Source: CAD feature listing. Evaluate the final solid. Frame: model axes, mm. Face numbers are marked on the shaded views. Round coordinates to 2 decimals unless told otherwise and drop trailing zeros. Order: outer loops, then holes, each group sorted by start corner. A loop starts at its lowest first (then second) coordinate and runs counter-clockwise, first axis right, second up. Notation, with made-up numbers: (-28, -17.75) -> (26, -17.75) arc R4 cw to (26, -10.75) -> close; hole circle Ø3 at (45, -23). An arc over 180 degrees is marked (long way). Write item = value, one per line. Start each with the question number.
(1) Cut plane C-C on x = 0. Return the cut outline in (y, z).
(2) Contact query for a flat-ended pin moving along its axis: pin 1 Ø1.6 at (x, y) = (0, -7.64) entering from -Z. Output: stop coordinate, or through.
(3) Ray query, line 1 (Y direction, x = 0, z = 1.9); line 2 (Y direction, x = -7, z = 0.8); line 3 (Y direction, x = 4, z = 1.45). Return the intervals inside material, ascending.
(4) Cut plane B-B on z = 1.7. Give the number of separate pieces and of enclosed holes in the cut face, then the cut area to 3 significant figures.
(5) Cut plane D-D on y = -7.64. Return the cut outline in (x, z).
(6) Cut plane A-A on y = 0. Return the cut outline in (x, z).
(7) Draft query along Y for the marked faces 1, 2, 3 and 4. Return one class per face: released by +Y, released by -Y, zero draft, split by the parting line, or undercut.
from build123d import *

# Parameters (mm, degrees)
SKETCH1_R              = 16
BOSS_EXTRUDE1_DEPTH    = 3
M1_6_CLEARANCE_HOLE1_D = 1.8
F_4_CLEARANCE_HOLE1_D  = 3.2639
F_2_CLEARANCE_HOLE1_D  = 2.4384


with BuildPart() as part:
    # Sketch1 → Boss-Extrude1 (new body)
    with BuildSketch(Plane.XY):
        Circle(SKETCH1_R)
    extrude(amount=BOSS_EXTRUDE1_DEPTH)

    # M1.6 Clearance Hole1 (through all)
    with Locations(Plane.XY.offset(3)):
        with Locations((-3.48, 7.64), (0, 7.64), (3.48, 7.64), (7.64, 3.48), (7.64, -3.48), (7.64, 0), (3.48, -7.64), (0, -7.64), (-3.48, -7.64), (-7.64, 0), (-7.64, -3.48), (-7.64, 3.48)):
            Hole(M1_6_CLEARANCE_HOLE1_D / 2)

    # #4 Clearance Hole1 (through all)
    with Locations(Plane.XY.offset(3)):
        with Locations((-13.09, 0), (13.09, 0)):
            Hole(F_4_CLEARANCE_HOLE1_D / 2)

    # #2 Clearance Hole1 (through all)
    with Locations(Plane.XY.offset(3)):
        with Locations((0, 0)):
            Hole(F_2_CLEARANCE_HOLE1_D / 2)


solid = part.part
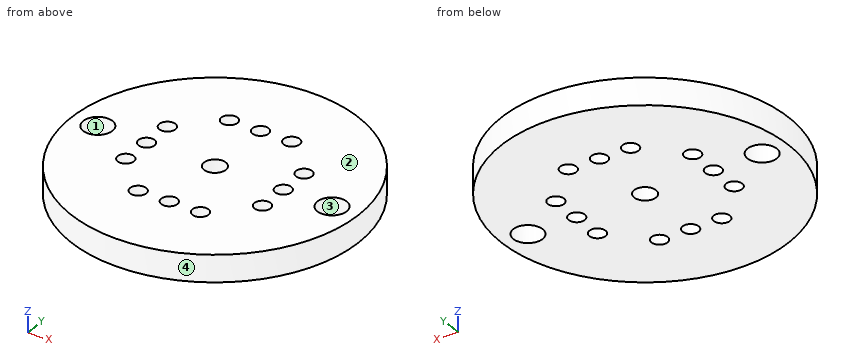
Evaluation:
q1.outline = (-16, 0) -> (-8.54, 0) -> (-8.54, 3) -> (-16, 3) -> close; (-6.74, 0) -> (-1.22, 0) -> (-1.22, 3) -> (-6.74, 3) -> close; (1.22, 0) -> (6.74, 0) -> (6.74, 3) -> (1.22, 3) -> close; (8.54, 0) -> (16, 0) -> (16, 3) -> (8.54, 3) -> close
q2.pin_1 = through
q3.line_1 = -16 to -8.54, -6.74 to -1.22, 1.22 to 6.74, 8.54 to 16
q3.line_2 = -14.39 to -4.11, -2.85 to -0.63, 0.63 to 2.85, 4.11 to 14.39
q3.line_3 = -15.49 to -8.37, -6.91 to 6.91, 8.37 to 15.49
q4.separate_pieces = 1
q4.enclosed_holes = 15
q4.area = 752 mm^2
q5.outline = (-14.06, 0) -> (-4.38, 0) -> (-4.38, 3) -> (-14.06, 3) -> close; (-2.58, 0) -> (-0.9, 0) -> (-0.9, 3) -> (-2.58, 3) -> close; (0.9, 0) -> (2.58, 0) -> (2.58, 3) -> (0.9, 3) -> close; (4.38, 0) -> (14.06, 0) -> (14.06, 3) -> (4.38, 3) -> close
q6.outline = (-16, 0) -> (-14.72, 0) -> (-14.72, 3) -> (-16, 3) -> close; (-11.46, 0) -> (-8.54, 0) -> (-8.54, 3) -> (-11.46, 3) -> close; (-6.74, 0) -> (-1.22, 0) -> (-1.22, 3) -> (-6.74, 3) -> close; (1.22, 0) -> (6.74, 0) -> (6.74, 3) -> (1.22, 3) -> close; (8.54, 0) -> (11.46, 0) -> (11.46, 3) -> (8.54, 3) -> close; (14.72, 0) -> (16, 0) -> (16, 3) -> (14.72, 3) -> close
q7.face_1 = undercut
q7.face_2 = zero draft
q7.face_3 = undercut
q7.face_4 = split by the parting line
